Could you check a few things on this model? Use its own coordinates, in mm. A direction names the side the tool comes from. Coordinates: 2 decimals unless noted, no trailing zeros. Order: outer loops, then holes, each group sorted by start corner. A loop starts at its lowest first (then second) coordinate and runs counter-clockwise, first axis right, second up. Notation, with made-up numbers: (-9, -14) - (9, -14) arc R14 cw to (9, -9) - close; hole circle Ø3 at (-3, -4.75). An arc over 180 degrees is marked (long way). One line per item, written item: value. Start each with the question number.
from build123d import *

# Parameters (mm, degrees)
BOSS_EXTRUDE1_DEPTH = 8.1
SKETCH3_R           = 3.268605963
CUT_EXTRUDE1_DEPTH  = 40


with BuildPart() as part:
    # Sketch1 → Revolve1 (revolve)
    with BuildSketch(Plane.XY, mode=Mode.PRIVATE) as revolve1_sk:
        Polygon((0, 0), (0, 31), (3.611174949, 31), (4.6, 29.2), (4.6, 18.1), (6.3, 18.1), (6.3, 10), (5, 10), (5, 0), align=None)
    revolve(revolve1_sk.sketch.rotate(Axis((0, 0, 0), (0, 1, 0)), 90), axis=Axis((0, 0, 0), (0, 1, 0)))

    # Sketch2 → Boss-Extrude1 (add)
    with BuildSketch(Plane(origin=(0, 18.1, 0), x_dir=(1, 0, 0), z_dir=(0, 1, 0))):
        Polygon((7.271508979, -0.636593264), (4.187060428, 5.979014867), (-3.08444855, 6.615608132), (-7.271508979, 0.636593264), (-4.187060428, -5.979014867), (3.08444855, -6.615608132), align=None)
    extrude(amount=-BOSS_EXTRUDE1_DEPTH)

    # Sketch3 → Cut-Extrude1 (cut)
    with BuildSketch(Plane(origin=(0, 31, 0), x_dir=(1, 0, 0), z_dir=(0, 1, 0))):
        with Locations(Location((0, 0, 0), (0, 0, 270))):
            Circle(SKETCH3_R)
    extrude(amount=-CUT_EXTRUDE1_DEPTH, mode=Mode.SUBTRACT)


solid = part.part
Q1. I want a section at B-B on y = 12.5. Please give me the cut outline in (x, z), then the cut area to 3 significant figures.
Q2. We'd pull the mould along Z, two halves only. Please class faces 4 (the cylindrical face through (-1.989, 15.717, -2.594)), 5 (the cylindrical face through (0, 5, 5)), 6 (the flat face through (5.751, 14.107, -2.625)), 7 (the flat face through (1, 0, -3.3)): +Z half, -Z half, draft (parallel to the pull), parting line (faces both ways), or undercut.
Q3. I'm going to push flat-ended pins straight in: pin 1 (1 mm diameter, centred on x = -2.5, y = 15.5, fed in from +Z); pin 2 (2 mm diameter, centred on x = -2, z = -1.5, fed in from +Y); pin 3 (1 mm diameter, centred on x = -5.5, z = 2.5, fed in from +Y); pin 4 (4 mm diameter, centred on x = 5.5, y = 26, fed in from +Z). Where does each tip first touch, or does it pass through?
Q4. I want a section at A-A on x = 0. Please give me the cut outline in (y, z).
Q5. I want a section at C-C on z = 0. Please give me the cut outline in (x, y), then the cut area to 3 significant figures.
Q6. I want a section at D-D on z = -5.5. Please give me the cut outline in (x, y).
Q7. Which directions (+Z, -Z, +X, -X, +Y, -Y) give clear straight access to the entire face, cutting with the end or side of a thin tool? Please do faces 1 (the flat face through (-5.751, 14.107, 2.625)), 2 (the cylindrical face through (2.8, 23.57, 3.65)), 3 (the flat face through (-2, 10, 5)).
Q8. If I drill on L1, parallel to X at y = 7.5, z = 0; L2, parallel to X at y = 19, z = 0; L3, parallel to Y at x = -3.25, z = 3.5, over which ranges is the centre line in solid material (lowest first)?
Values follow:
1. outline: (-7.27, -0.64) - (-3.08, -6.62) - (4.19, -5.98) - (7.27, 0.64) - (3.08, 6.62) - (-4.19, 5.98) - close; hole circle Ø6.54 at (0, 0)
1. area: 105 mm^2
2. face 4: undercut
2. face 5: parting line
2. face 6: -Z half
2. face 7: draft
3. pin 1: stops at z = 6.17
3. pin 2: stops at y = 31
3. pin 3: stops at y = 18.1
3. pin 4: stops at z = 2.98
4. outline: (0, -5) - (10, -5) - (10, -6.35) - (18.1, -6.35) - (18.1, -4.6) - (29.2, -4.6) - (31, -3.61) - (31, -3.27) - (0, -3.27) - close; (0, 3.27) - (31, 3.27) - (31, 3.61) - (29.2, 4.6) - (18.1, 4.6) - (18.1, 6.35) - (10, 6.35) - (10, 5) - (0, 5) - close
5. outline: (-6.97, 10) - (-5, 10) - (-5, 0) - (-3.27, 0) - (-3.27, 31) - (-3.61, 31) - (-4.6, 29.2) - (-4.6, 18.1) - (-6.97, 18.1) - close; (3.27, 0) - (5, 0) - (5, 10) - (6.97, 10) - (6.97, 18.1) - (4.6, 18.1) - (4.6, 29.2) - (3.61, 31) - (3.27, 31) - close
5. area: 127 mm^2
6. outline: (-3.87, 10) - (4.41, 10) - (4.41, 18.1) - (-3.87, 18.1) - close
7. face 1: +Z, -X, +Y, -Y
7. face 2: +Y
7. face 3: -Y
8. L1: x = -5 to -3.27, 3.27 to 5
8. L2: x = -4.6 to -3.27, 3.27 to 4.6
8. L3: y = 0 to 18.1
